The drawing under review shows one solid part. Ordinate dimensions are in mm from its lowest x, y, z. A direction names the side the tool comes from. Give positions to 0.01 mm unless a question says otherwise; leave off trailing zeros. Order: outer loops, then holes, each group sorted by start corner. A loop starts at its lowest first (then second) coordinate and runs counter-clockwise, first axis right, second up. Notation, with made-up numbers: (18.25, 25) - (36.25, 25) arc R12 cw to (36.25, 47) - close; hole circle Ø11 at (74.25, -8.5). An arc over 180 degrees is marked (long way). Answer as a JSON object with one key per item and string values. Group by question number.
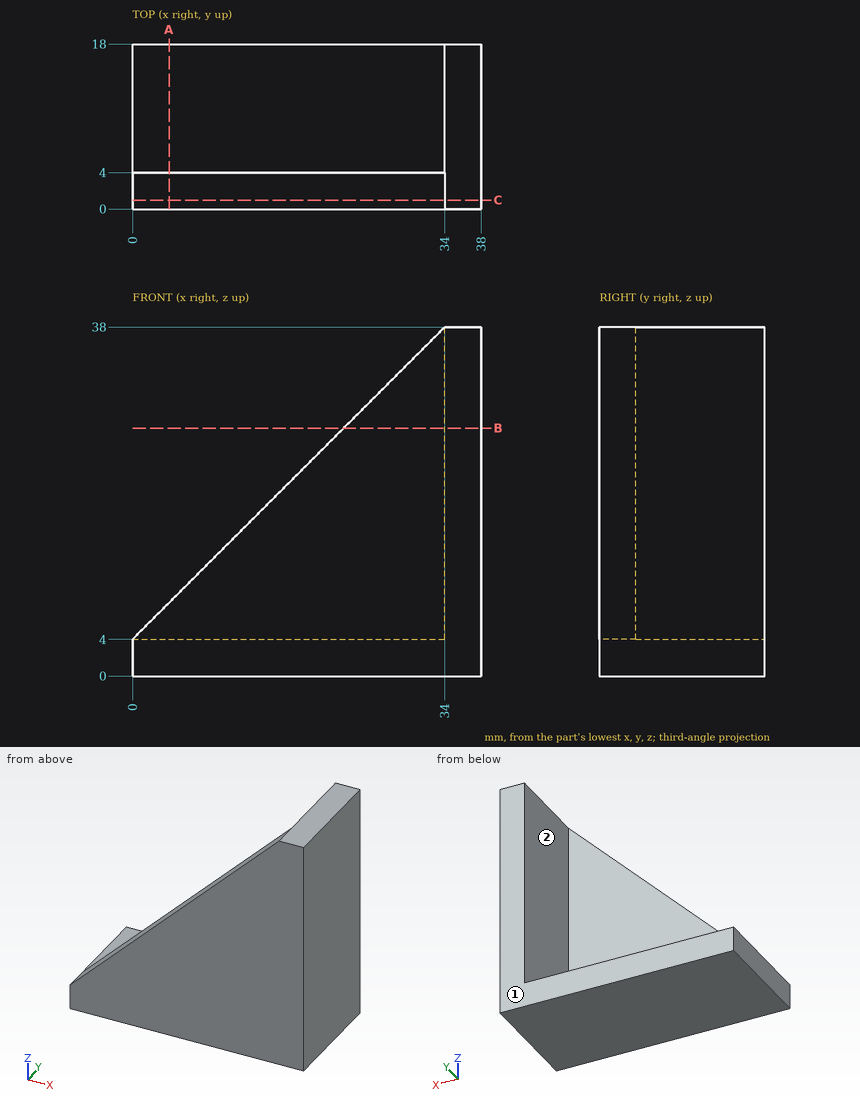
1) For line 1 (X direction, y = 10, z = 27); line 2 (Y direction, x = 20, z = 10.5); line 3 (X direction, y = 3, z = 8), list the stretches that pass through material, from the lowest coordinate up.
2) Consider section A-A (x = 4). Give the boundary of the cut face in (y, z), plus the area to 3 significant figures.
3) For pin 1 (10 mm diameter, centred on x = 13.5, z = 6, fed in from +Y); pin 2 (1 mm diameter, centred on y = 8.5, z = 33.5, fed in from -X); pin 3 (1.5 mm diameter, centred on x = 16, y = 6.5, fed in from +Z); pin 4 (1.5 mm diameter, centred on x = 16.5, y = 3.5, fed in from +Z), all flat-tipped, find the tip position at first contact; note any pin that passes through.
4) Consider section B-B (z = 27). Give the boundary of the cut face in (x, y), plus the area to 3 significant figures.
5) For the marked faces 1 and 2, list the 3-axis set-ups (+Z, -Z, +X, -X, +Y, -Y) from which the entire face can be reached by the end or side of a thin tool; tool diameter is ignored.
6) Consider section C-C (y = 1). Give the boundary of the cut face in (x, z).
Result set:
{
 "1": {"line 1": "x = 34 to 38", "line 2": "y = 0 to 4", "line 3": "x = 4 to 38"},
 "2": {"outline": "(0, 0) - (18, 0) - (18, 4) - (4, 4) - (4, 8) - (0, 8) - close", "area": "88.0 mm2"},
 "3": {"pin 1": "stops at y = 18", "pin 2": "stops at x = 34", "pin 3": "stops at z = 4", "pin 4": "stops at z = 21.25"},
 "4": {"outline": "(23, 0) - (38, 0) - (38, 18) - (34, 18) - (34, 4) - (23, 4) - close", "area": "116 mm2"},
 "5": {"face 1": "+Z, -Z, +X, -X, +Y", "face 2": "+Z, -X, +Y"},
 "6": {"outline": "(0, 0) - (38, 0) - (38, 38) - (34, 38) - (0, 4) - close"}
}
